```python
from build123d import *

# Parameters (mm, degrees)
MODEL_R             = 1
BOSS_EXTRUDE1_DEPTH = 3
CUT_EXTRUDE1_START  = 3
MODEL_3_R           = 1.8
CUT_EXTRUDE1_DEPTH  = 1.5
SKETCH3_W           = 3.410478587
SKETCH3_H           = 49.945504098
SKETCH3_W_2         = 6.648180457
SKETCH3_H_2         = 47.210710856
CUT_EXTRUDE2_DEPTH  = 5
SKETCH4_R           = 3.544423748
SKETCH4_R_2         = 2.369129831
BOSS_EXTRUDE2_DEPTH = 7


with BuildPart() as part:
    # Model → Boss-Extrude1 (new body)
    with BuildSketch(Plane.XY):
        Polygon((0, -78), (123, -78.361463573), (123, -0.361463573), (0, 0), align=None)
        with Locations((4.834975253, -4.704019458)):
            Circle(MODEL_R, mode=Mode.SUBTRACT)
        with Locations((46.124975253, -19.448037489)):
            Circle(MODEL_R, mode=Mode.SUBTRACT)
        with Locations((42.286307754, -39.29983525)):
            Circle(MODEL_R, mode=Mode.SUBTRACT)
        with Locations((4.834975253, -35.973037489)):
            Circle(MODEL_R, mode=Mode.SUBTRACT)
        with Locations((85.542975253, -4.704019458)):
            Circle(MODEL_R, mode=Mode.SUBTRACT)
        with Locations((5.334975253, -70.100370509)):
            Circle(MODEL_R, mode=Mode.SUBTRACT)
        with Locations((112.441999555, -70.100370509)):
            Circle(MODEL_R, mode=Mode.SUBTRACT)
        with BuildLine():
            Line((9.144975253, -2.923037489), (22.144975253, -2.923037489))
            ThreePointArc((22.144975253, -2.923037489), (22.498528643, -3.069484099), (22.644975253, -3.423037489))
            Line((22.644975253, -3.423037489), (22.644975253, -16.423037489))
            ThreePointArc((22.644975253, -16.423037489), (22.498528643, -16.77659088), (22.144975253, -16.923037489))
            Line((22.144975253, -16.923037489), (9.144975253, -16.923037489))
            ThreePointArc((9.144975253, -16.923037489), (8.791421862, -16.77659088), (8.644975253, -16.423037489))
            Line((8.644975253, -16.423037489), (8.644975253, -3.423037489))
            ThreePointArc((8.644975253, -3.423037489), (8.791421862, -3.069484099), (9.144975253, -2.923037489))
        make_face(mode=Mode.SUBTRACT)
        with BuildLine():
            Line((28.194975253, -2.923037489), (41.194975253, -2.923037489))
            ThreePointArc((41.194975253, -2.923037489), (41.548528643, -3.069484099), (41.694975253, -3.423037489))
            Line((41.694975253, -3.423037489), (41.694975253, -16.423037489))
            ThreePointArc((41.694975253, -16.423037489), (41.548528643, -16.77659088), (41.194975253, -16.923037489))
            Line((41.194975253, -16.923037489), (28.194975253, -16.923037489))
            ThreePointArc((28.194975253, -16.923037489), (27.841421862, -16.77659088), (27.694975253, -16.423037489))
            Line((27.694975253, -16.423037489), (27.694975253, -3.423037489))
            ThreePointArc((27.694975253, -3.423037489), (27.841421862, -3.069484099), (28.194975253, -2.923037489))
        make_face(mode=Mode.SUBTRACT)
        with BuildLine():
            Line((47.244975253, -2.923037489), (60.244975253, -2.923037489))
            ThreePointArc((60.244975253, -2.923037489), (60.598528643, -3.069484099), (60.744975253, -3.423037489))
            Line((60.744975253, -3.423037489), (60.744975253, -16.423037489))
            ThreePointArc((60.744975253, -16.423037489), (60.598528643, -16.77659088), (60.244975253, -16.923037489))
            Line((60.244975253, -16.923037489), (47.244975253, -16.923037489))
            ThreePointArc((47.244975253, -16.923037489), (46.891421862, -16.77659088), (46.744975253, -16.423037489))
            Line((46.744975253, -16.423037489), (46.744975253, -3.423037489))
            ThreePointArc((46.744975253, -3.423037489), (46.891421862, -3.069484099), (47.244975253, -2.923037489))
        make_face(mode=Mode.SUBTRACT)
        with BuildLine():
            Line((66.294975253, -2.923037489), (79.294975253, -2.923037489))
            ThreePointArc((79.294975253, -2.923037489), (79.648528643, -3.069484099), (79.794975253, -3.423037489))
            Line((79.794975253, -3.423037489), (79.794975253, -16.423037489))
            ThreePointArc((79.794975253, -16.423037489), (79.648528643, -16.77659088), (79.294975253, -16.923037489))
            Line((79.294975253, -16.923037489), (66.294975253, -16.923037489))
            ThreePointArc((66.294975253, -16.923037489), (65.941421862, -16.77659088), (65.794975253, -16.423037489))
            Line((65.794975253, -16.423037489), (65.794975253, -3.423037489))
            ThreePointArc((65.794975253, -3.423037489), (65.941421862, -3.069484099), (66.294975253, -2.923037489))
        make_face(mode=Mode.SUBTRACT)
        with BuildLine():
            Line((12.954975253, -21.973037489), (25.954975253, -21.973037489))
            ThreePointArc((25.954975253, -21.973037489), (26.308528643, -22.119484099), (26.454975253, -22.473037489))
            Line((26.454975253, -22.473037489), (26.454975253, -35.473037489))
            ThreePointArc((26.454975253, -35.473037489), (26.308528643, -35.82659088), (25.954975253, -35.973037489))
            Line((25.954975253, -35.973037489), (12.954975253, -35.973037489))
            ThreePointArc((12.954975253, -35.973037489), (12.601421862, -35.82659088), (12.454975253, -35.473037489))
            Line((12.454975253, -35.473037489), (12.454975253, -22.473037489))
            ThreePointArc((12.454975253, -22.473037489), (12.601421862, -22.119484099), (12.954975253, -21.973037489))
        make_face(mode=Mode.SUBTRACT)
        with BuildLine():
            Line((32.004975253, -21.973037489), (45.004975253, -21.973037489))
            ThreePointArc((45.004975253, -21.973037489), (45.358528643, -22.119484099), (45.504975253, -22.473037489))
            Line((45.504975253, -22.473037489), (45.504975253, -35.473037489))
            ThreePointArc((45.504975253, -35.473037489), (45.358528643, -35.82659088), (45.004975253, -35.973037489))
            Line((45.004975253, -35.973037489), (32.004975253, -35.973037489))
            ThreePointArc((32.004975253, -35.973037489), (31.651421862, -35.82659088), (31.504975253, -35.473037489))
            Line((31.504975253, -35.473037489), (31.504975253, -22.473037489))
            ThreePointArc((31.504975253, -22.473037489), (31.651421862, -22.119484099), (32.004975253, -21.973037489))
        make_face(mode=Mode.SUBTRACT)
        with BuildLine():
            Line((51.054975253, -21.973037489), (64.054975253, -21.973037489))
            ThreePointArc((64.054975253, -21.973037489), (64.408528643, -22.119484099), (64.554975253, -22.473037489))
            Line((64.554975253, -22.473037489), (64.554975253, -35.473037489))
            ThreePointArc((64.554975253, -35.473037489), (64.408528643, -35.82659088), (64.054975253, -35.973037489))
            Line((64.054975253, -35.973037489), (51.054975253, -35.973037489))
            ThreePointArc((51.054975253, -35.973037489), (50.701421862, -35.82659088), (50.554975253, -35.473037489))
            Line((50.554975253, -35.473037489), (50.554975253, -22.473037489))
            ThreePointArc((50.554975253, -22.473037489), (50.701421862, -22.119484099), (51.054975253, -21.973037489))
        make_face(mode=Mode.SUBTRACT)
        with BuildLine():
            Line((70.104975253, -21.973037489), (83.104975253, -21.973037489))
            ThreePointArc((83.104975253, -21.973037489), (83.458528643, -22.119484099), (83.604975253, -22.473037489))
            Line((83.604975253, -22.473037489), (83.604975253, -35.473037489))
            ThreePointArc((83.604975253, -35.473037489), (83.458528643, -35.82659088), (83.104975253, -35.973037489))
            Line((83.104975253, -35.973037489), (70.104975253, -35.973037489))
            ThreePointArc((70.104975253, -35.973037489), (69.751421862, -35.82659088), (69.604975253, -35.473037489))
            Line((69.604975253, -35.473037489), (69.604975253, -22.473037489))
            ThreePointArc((69.604975253, -22.473037489), (69.751421862, -22.119484099), (70.104975253, -21.973037489))
        make_face(mode=Mode.SUBTRACT)
        with BuildLine():
            Line((5.334975253, -41.023037489), (18.334975253, -41.023037489))
            ThreePointArc((18.334975253, -41.023037489), (18.688528643, -41.169484099), (18.834975253, -41.523037489))
            Line((18.834975253, -41.523037489), (18.834975253, -54.523037489))
            ThreePointArc((18.834975253, -54.523037489), (18.688528643, -54.87659088), (18.334975253, -55.023037489))
            Line((18.334975253, -55.023037489), (5.334975253, -55.023037489))
            ThreePointArc((5.334975253, -55.023037489), (4.981421862, -54.87659088), (4.834975253, -54.523037489))
            Line((4.834975253, -54.523037489), (4.834975253, -41.523037489))
            ThreePointArc((4.834975253, -41.523037489), (4.981421862, -41.169484099), (5.334975253, -41.023037489))
        make_face(mode=Mode.SUBTRACT)
        with BuildLine():
            Line((26.289975253, -41.023037489), (39.289975253, -41.023037489))
            ThreePointArc((39.289975253, -41.023037489), (39.643528643, -41.169484099), (39.789975253, -41.523037489))
            Line((39.789975253, -41.523037489), (39.789975253, -54.523037489))
            ThreePointArc((39.789975253, -54.523037489), (39.643528643, -54.87659088), (39.289975253, -55.023037489))
            Line((39.289975253, -55.023037489), (26.289975253, -55.023037489))
            ThreePointArc((26.289975253, -55.023037489), (25.936421862, -54.87659088), (25.789975253, -54.523037489))
            Line((25.789975253, -54.523037489), (25.789975253, -41.523037489))
            ThreePointArc((25.789975253, -41.523037489), (25.936421862, -41.169484099), (26.289975253, -41.023037489))
        make_face(mode=Mode.SUBTRACT)
        with BuildLine():
            Line((45.339975253, -41.023037489), (58.339975253, -41.023037489))
            ThreePointArc((58.339975253, -41.023037489), (58.693528643, -41.169484099), (58.839975253, -41.523037489))
            Line((58.839975253, -41.523037489), (58.839975253, -54.523037489))
            ThreePointArc((58.839975253, -54.523037489), (58.693528643, -54.87659088), (58.339975253, -55.023037489))
            Line((58.339975253, -55.023037489), (45.339975253, -55.023037489))
            ThreePointArc((45.339975253, -55.023037489), (44.986421862, -54.87659088), (44.839975253, -54.523037489))
            Line((44.839975253, -54.523037489), (44.839975253, -41.523037489))
            ThreePointArc((44.839975253, -41.523037489), (44.986421862, -41.169484099), (45.339975253, -41.023037489))
        make_face(mode=Mode.SUBTRACT)
        with BuildLine():
            Line((64.389975253, -41.023037489), (77.389975253, -41.023037489))
            ThreePointArc((77.389975253, -41.023037489), (77.743528643, -41.169484099), (77.889975253, -41.523037489))
            Line((77.889975253, -41.523037489), (77.889975253, -54.523037489))
            ThreePointArc((77.889975253, -54.523037489), (77.743528643, -54.87659088), (77.389975253, -55.023037489))
            Line((77.389975253, -55.023037489), (64.389975253, -55.023037489))
            ThreePointArc((64.389975253, -55.023037489), (64.036421862, -54.87659088), (63.889975253, -54.523037489))
            Line((63.889975253, -54.523037489), (63.889975253, -41.523037489))
            ThreePointArc((63.889975253, -41.523037489), (64.036421862, -41.169484099), (64.389975253, -41.023037489))
        make_face(mode=Mode.SUBTRACT)
        with BuildLine():
            Line((70.104975253, -60.073037489), (83.104975253, -60.073037489))
            ThreePointArc((83.104975253, -60.073037489), (83.458528643, -60.219484099), (83.604975253, -60.573037489))
            Line((83.604975253, -60.573037489), (83.604975253, -73.573037489))
            ThreePointArc((83.604975253, -73.573037489), (83.458528643, -73.92659088), (83.104975253, -74.073037489))
            Line((83.104975253, -74.073037489), (70.104975253, -74.073037489))
            ThreePointArc((70.104975253, -74.073037489), (69.751421862, -73.92659088), (69.604975253, -73.573037489))
            Line((69.604975253, -73.573037489), (69.604975253, -60.573037489))
            ThreePointArc((69.604975253, -60.573037489), (69.751421862, -60.219484099), (70.104975253, -60.073037489))
        make_face(mode=Mode.SUBTRACT)
    extrude(amount=BOSS_EXTRUDE1_DEPTH)

    # Model<3> → Cut-Extrude1 (cut)
    with BuildSketch(Plane.XY.offset(CUT_EXTRUDE1_START)):
        with Locations((85.542975253, -4.704019458)):
            Circle(MODEL_3_R)
        with Locations((4.834975253, -4.704019458)):
            Circle(MODEL_3_R)
        with Locations((46.124975253, -19.448037489)):
            Circle(MODEL_3_R)
        with Locations((42.286307754, -39.29983525)):
            Circle(MODEL_3_R)
        with Locations((4.834975253, -35.973037489)):
            Circle(MODEL_3_R)
        with Locations((5.334975253, -70.100370509)):
            Circle(MODEL_3_R)
        with Locations((112.441999555, -70.100370509)):
            Circle(MODEL_3_R)
    extrude(amount=-CUT_EXTRUDE1_DEPTH, mode=Mode.SUBTRACT)

    # Sketch3 → Cut-Extrude2 (cut)
    with BuildSketch(Plane.XY.offset(3)):
        with Locations((92.139427294, -25.238513551)):
            Rectangle(SKETCH3_W, SKETCH3_H)
        with Locations((119.675909772, -23.947281806)):
            Rectangle(SKETCH3_W_2, SKETCH3_H_2)
    extrude(amount=-CUT_EXTRUDE2_DEPTH, mode=Mode.SUBTRACT)

    # Sketch4 → Boss-Extrude2 (add)
    with BuildSketch(Plane.XY):
        with Locations((104.757578873, -16.130439743)):
            Circle(SKETCH4_R)
        with Locations((104.757578873, -16.130439743)):
            Circle(SKETCH4_R_2, mode=Mode.SUBTRACT)
    extrude(amount=-BOSS_EXTRUDE2_DEPTH)


solid = part.part
```
The model under review builds one solid part; all positions refer to its coordinate system, in mm. A direction names the side the tool comes from. Round coordinates to 2 decimals unless told otherwise and drop trailing zeros. Order: outer loops, then holes, each group sorted by start corner. A loop starts at its lowest first (then second) coordinate and runs counter-clockwise, first axis right, second up. Notation, with made-up numbers: (-28, 14) -> (-13, 14) arc R16 cw to (-13, 42) -> close; hole circle Ø9 at (79, -33). An arc over 180 degrees is marked (long way). One line per item, written item: value. Start each with the question number.
Q1. Wall thickness on line 1 (X direction, y = -49, z = 0.5); line 2 (X direction, y = -20.5, z = 0.25); line 3 (X direction, y = -62.5, z = 1): over which ranges is each line inside the solid? List them lowest first.
Q2. Take a section at A-A (y = -64.5). Write out the cut boundary in (x, z), and give its area (3 significant figures).
Q3. Machinability: for faces 1 (the face through (27.695, -10, 1)), 2 (the face through (61, -47, 3)), 3 (the face through (6, -5, 1.5)), which of the approach directions +Z, -Z, +X, -X, +Y, -Y give a long, thin tool a straight path to every point of the face, cutting with its end or side? Answer none if there is none.
Q4. Clearance check with flat-ended pins moving along their axes: pin 1 Ø2.5 at (y, z) = (-21, 1.5) entering from +X; pin 2 Ø1.5 at (x, z) = (16.5, 2) entering from +Y; pin 3 Ø3.5 at (x, z) = (78.5, 1.5) entering from +Y. State where each tip first meets the part, or that it passes through.
Q5. Mouldability with a two-part tool opening along X and no side actions: class faces 4 (the face through (0, -38, 1)), 5 (the face through (123, -63, 1)), 6 (the face through (71, -41.023, 1)) as released by +X, released by -X, zero draft, split by the parting line, or undercut.
Q6. Take a section at B-B (x = 24.5). Write out the cut boundary in (y, z).
Q7. Take a section at C-C (z = -5.5). Write out the cut boundary in (x, y).
Reported:
1. line 1: x = 0 to 4.83, 18.83 to 25.79, 39.79 to 44.84, 58.84 to 63.89, 77.89 to 90.43, 93.84 to 123
1. line 2: x = 0 to 90.43, 93.84 to 116.35
1. line 3: x = 0 to 69.6, 83.6 to 123
2. outline: (0, 0) -> (69.6, 0) -> (69.6, 3) -> (0, 3) -> close; (83.6, 0) -> (123, 0) -> (123, 3) -> (83.6, 3) -> close
2. area: 327 mm2
3. face 1: +Z, -Z
3. face 2: +Z, +X, -X, +Y, -Y
3. face 3: +Z
4. pin 1: stops at x = 116.35
4. pin 2: stops at y = -0.05
4. pin 3: stops at y = -0.23
5. face 4: released by -X
5. face 5: released by +X
5. face 6: undercut
6. outline: (-78.07, 0) -> (-35.97, 0) -> (-35.97, 3) -> (-78.07, 3) -> close; (-21.97, 0) -> (-0.07, 0) -> (-0.07, 3) -> (-21.97, 3) -> close
7. outline: circle Ø7.09 at (104.76, -16.13); hole circle Ø4.74 at (104.76, -16.13)
